from build123d import *

# Parameters (mm, degrees)
BOSS_EXTRUDE1_DEPTH = 38.1
SKETCH2_R           = 12.065
CUT_EXTRUDE1_DEPTH  = 25.4
SKETCH7_R           = 12.065
CUT_EXTRUDE2_DEPTH  = 25.4
SKETCH8_W           = 26.289
SKETCH8_H           = 26.289
BOSS_EXTRUDE2_DEPTH = 8.89


with BuildPart() as part:
    # Sketch1 → Boss-Extrude1 (new body)
    with BuildSketch(Plane(origin=(0, 0, 0), x_dir=(1, 0, 0), z_dir=(0, 1, 0))):
        with BuildLine():
            Line((-8.394951703, 35.720764917), (16.107614613, 27.828435078))
            ThreePointArc((16.107614613, 27.828435078), (18.03059142, 27.370657964), (20.001310729, 27.216823331))
            Line((20.001310729, 27.216823331), (122.238689271, 27.216823331))
            ThreePointArc((122.238689271, 27.216823331), (124.20940858, 27.370657964), (126.132385387, 27.828435078))
            Line((126.132385387, 27.828435078), (150.634951703, 35.720764917))
            ThreePointArc((150.634951703, 35.720764917), (157.509150211, 35.977683688), (163.508903941, 32.612632786))
            Line((163.508903941, 32.612632786), (184.96230509, 11.159231637))
            Line((184.96230509, 11.159231637), (158.021536726, -15.781536726))
            Line((158.021536726, -15.781536726), (142.24, 0))
            Line((142.24, 0), (127.676821583, 11.356327171))
            ThreePointArc((127.676821583, 11.356327171), (123.996342172, 13.351360126), (119.867179962, 14.041363479))
            Line((119.867179962, 14.041363479), (22.372820038, 14.041363479))
            ThreePointArc((22.372820038, 14.041363479), (18.243657828, 13.351360126), (14.563178417, 11.356327171))
            Line((14.563178417, 11.356327171), (0, 0))
            Line((0, 0), (-15.781536726, -15.781536726))
            Line((-15.781536726, -15.781536726), (-42.72230509, 11.159231637))
            Line((-42.72230509, 11.159231637), (-21.268903941, 32.612632786))
            ThreePointArc((-21.268903941, 32.612632786), (-15.269150211, 35.977683688), (-8.394951703, 35.720764917))
        make_face()
    extrude(amount=BOSS_EXTRUDE1_DEPTH)

    # Sketch2 → Cut-Extrude1 (cut)
    with BuildSketch(Plane(origin=(-15.781536726, 0, 15.781536726), x_dir=(0.7071067811865477, 0, 0.7071067811865475), z_dir=(-0.7071067811865475, 0, 0.7071067811865477))):
        with Locations((-19.05, 19.05)):
            Circle(SKETCH2_R)
    extrude(amount=-CUT_EXTRUDE1_DEPTH, mode=Mode.SUBTRACT)

    # Sketch7 → Cut-Extrude2 (cut)
    with BuildSketch(Plane(origin=(86.901536726, 0, 86.901536726), x_dir=(0.7071067811865472, 0, -0.7071067811865478), z_dir=(0.7071067811865478, 0, 0.7071067811865472))):
        with Locations((119.628868556, 19.05)):
            Circle(SKETCH7_R)
    extrude(amount=-CUT_EXTRUDE2_DEPTH, mode=Mode.SUBTRACT)

    # Sketch8 → Boss-Extrude2 (add)
    with BuildSketch(Plane.XY.offset(-14.041363479)):
        with Locations((71.12, 13.1445)):
            Rectangle(SKETCH8_W, SKETCH8_H)
    extrude(amount=BOSS_EXTRUDE2_DEPTH)


solid = part.part
The listing builds one solid part. Answer for the finished solid, in the listing's coordinates (mm). A direction names the side the tool comes from. Coordinates: 2 decimals unless noted, no trailing zeros. Loops run counter-clockwise (first coordinate to the right, second up) from the corner with the lowest first, then second, coordinate; pieces in that order, holes last. Notation, with made-up numbers: (-2, 81.5) -> (16, 81.5) arc R5 ccw to (16, 89.5) -> close; hole circle Ø8 at (-27.5, 50.5). An arc over 180 degrees is marked (long way). Answer in a Markdown table with one row per item. Add a question column.
1. For faces 1 (the flat face through (153.41, 19.22, -15.53)), 2 (the flat face through (84.264, 13, -10)), 3 (the flat face through (3.68, 18.78, -31.83)), determine the directions among +Z, -Z, +X, -X, +Y, -Y from which every point of the face is accessible in a straight line to the end or side of a thin tool.
2. Flat-ended cylindrical pins translate along their axes: P1, Ø8, axis at x = 68, y = 14.5, coming from the +Z side; P2, Ø12, axis at x = 56, z = -5.5, coming from the -Y side; P3, Ø4.5, axis at y = 8, z = -9.5, coming from the -X side; P4, Ø1, axis at y = 20, z = -28, coming from the +X side. Find the tip coordinate at first contact, or state that the pin passes through.
3. The part is cut by section B-B, the plane x = 60. Write down the section's boundary in (y, z).
4. The part is cut by section A-A, the plane z = 13. Write down the section's boundary in (x, y).
5. Consider line 1 (X direction, y = 13, z = -22); line 2 (Z direction, x = 70, y = 35); line 3 (X direction, y = 22, z = 1). Determine where each line is inside the solid, lowest interval first. Write a range as [from, to].
6. Determine the mould class of faces 4 (the flat face through (73, 38.1, -16)), 5 (the flat face through (-11.41, 19.22, -15.77)), 6 (the flat face through (174.085, 18.783, -22.036)) for opening direction X: +X half, -X half, draft (parallel to the pull), parting line (faces both ways), or undercut.
7. The part is cut by section D-D, the plane x = 4. Write down the section's boundary in (y, z).
Answer below:
| question | item | result |
|---|---|---|
| 1 | face 1 | none |
| 1 | face 2 | +Z, +Y, -Y |
| 1 | face 3 | -Z, +Y, -Y |
| 2 | P1 | z = -5.15 |
| 2 | P2 | y = 0 |
| 2 | P3 | x = -42.72 |
| 2 | P4 | x = 168.62 |
| 3 | outline | (0, -27.22) -> (38.1, -27.22) -> (38.1, -14.04) -> (26.29, -14.04) -> (26.29, -5.15) -> (0, -5.15) -> close |
| 4 | outline | (-18.56, 0) -> (-13, 0) -> (-13, 38.1) -> (-18.56, 38.1) -> close; (155.24, 0) -> (160.8, 0) -> (160.8, 38.1) -> (155.24, 38.1) -> close |
| 5 | line 1 | [-31.88, -19.7], [-17.64, 159.88], [161.94, 174.12] |
| 5 | line 2 | [-27.22, -14.04] |
| 5 | line 3 | [-11.4, -1], [143.24, 153.64] |
| 6 | face 4 | draft |
| 6 | face 5 | undercut |
| 6 | face 6 | +X half |
| 7 | outline | (0, -31.73) -> (38.1, -31.73) -> (38.1, -3.12) -> (0, -3.12) -> close |
